Verification items for the finished model (mm, model axes). Round coordinates to 2 decimals unless told otherwise and drop trailing zeros. Write each loop counter-clockwise with the first axis right and the second up, starting at its lowest first coordinate (ties: lowest second). Pieces come first, ordered by that corner, then holes. Notation, with made-up numbers: (53.5, -13) - (81.5, -13) arc R17 cw to (81.5, 17) - close; hole circle Ø6 at (-3.75, 84). An arc over 180 degrees is marked (long way). Answer as a JSON object with one key per item and string values.
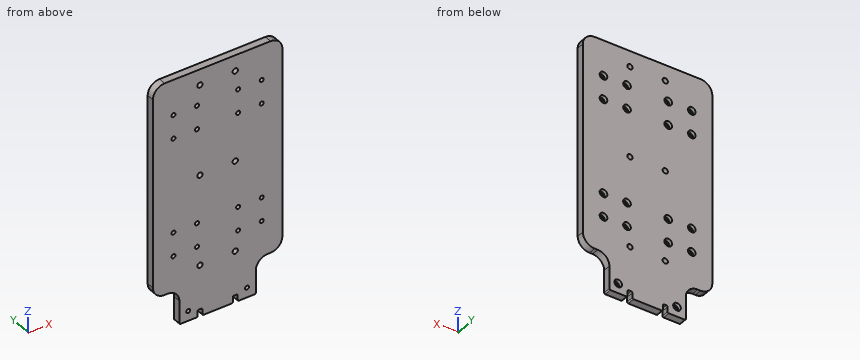
```python
from build123d import *

# Parameters (mm, degrees)
SKETCH1_W                      = 110
SKETCH1_H                      = 180
BOSS_EXTRUDE1_DEPTH            = 6.35
CBORE_START                    = 3.35
CBORE_FOR_M3_SHCS2_OUTLINE_R   = 3.25
CBORE_FOR_M3_SHCS2_DEPTH       = 3
CBORE_FOR_M3_SHCS2_2_OUTLINE_R = 1.7
CBORE_FOR_M3_SHCS2_2_DEPTH     = 3.35
M4_CLEARANCE_HOLE1_D           = 4.5
SKETCH6_W                      = 65
SKETCH6_H                      = 6.35
BOSS_EXTRUDE2_DEPTH            = 30
CBORE_FOR_M3_SHCS1_D           = 3.4
CBORE_FOR_M3_SHCS1_CBORE_D     = 6.5
CBORE_FOR_M3_SHCS1_CBORE_DEPTH = 3
FILLET2_R                      = 10
FILLET3_R                      = 10
SKETCH9_W                      = 4
SKETCH9_H                      = 6
CUT_EXTRUDE1_DEPTH             = 212.045782948
FILLET4_R                      = 1
FILLET5_R                      = 1
FILLET6_R                      = 1


# Read off the part's stored shape, not the designer's step: CBORE for M3 SHCS2
with BuildPart() as part:
    # Sketch1 → Boss-Extrude1 (new body)
    with BuildSketch(Plane(origin=(0, 0, 0), x_dir=(1, 0, 0), z_dir=(0, 1, 0))):
        with Locations((55, -90)):
            Rectangle(SKETCH1_W, SKETCH1_H)
    extrude(amount=BOSS_EXTRUDE1_DEPTH)

    # CBORE for M3 SHCS2 outline → CBORE for M3 SHCS2 (cut)
    with BuildSketch(Plane(origin=(0, 0, 0), x_dir=(1, 0, 0), z_dir=(0, 1, 0)).offset(CBORE_START)):
        with Locations((37.5, -150)):
            Circle(CBORE_FOR_M3_SHCS2_OUTLINE_R)
        with Locations((37.5, -130)):
            Circle(CBORE_FOR_M3_SHCS2_OUTLINE_R)
        with Locations((17.5, -130)):
            Circle(CBORE_FOR_M3_SHCS2_OUTLINE_R)
        with Locations((72.5, -150)):
            Circle(CBORE_FOR_M3_SHCS2_OUTLINE_R)
        with Locations((72.5, -130)):
            Circle(CBORE_FOR_M3_SHCS2_OUTLINE_R)
        with Locations((92.5, -130)):
            Circle(CBORE_FOR_M3_SHCS2_OUTLINE_R)
        with Locations((72.5, -30)):
            Circle(CBORE_FOR_M3_SHCS2_OUTLINE_R)
        with Locations((92.5, -50)):
            Circle(CBORE_FOR_M3_SHCS2_OUTLINE_R)
        with Locations((72.5, -50)):
            Circle(CBORE_FOR_M3_SHCS2_OUTLINE_R)
        with Locations((37.5, -30)):
            Circle(CBORE_FOR_M3_SHCS2_OUTLINE_R)
        with Locations((17.5, -50)):
            Circle(CBORE_FOR_M3_SHCS2_OUTLINE_R)
        with Locations((37.5, -50)):
            Circle(CBORE_FOR_M3_SHCS2_OUTLINE_R)
        with Locations((92.5, -150)):
            Circle(CBORE_FOR_M3_SHCS2_OUTLINE_R)
        with Locations((17.5, -30)):
            Circle(CBORE_FOR_M3_SHCS2_OUTLINE_R)
        with Locations((17.5, -150)):
            Circle(CBORE_FOR_M3_SHCS2_OUTLINE_R)
        with Locations((92.5, -30)):
            Circle(CBORE_FOR_M3_SHCS2_OUTLINE_R)
    extrude(amount=CBORE_FOR_M3_SHCS2_DEPTH, mode=Mode.SUBTRACT)

    # CBORE for M3 SHCS2 2 outline → CBORE for M3 SHCS2 2 (cut)
    with BuildSketch(Plane(origin=(0, 0, 0), x_dir=(1, 0, 0), z_dir=(0, 1, 0))):
        with Locations((37.5, -150)):
            Circle(CBORE_FOR_M3_SHCS2_2_OUTLINE_R)
        with Locations((37.5, -130)):
            Circle(CBORE_FOR_M3_SHCS2_2_OUTLINE_R)
        with Locations((17.5, -130)):
            Circle(CBORE_FOR_M3_SHCS2_2_OUTLINE_R)
        with Locations((72.5, -150)):
            Circle(CBORE_FOR_M3_SHCS2_2_OUTLINE_R)
        with Locations((72.5, -130)):
            Circle(CBORE_FOR_M3_SHCS2_2_OUTLINE_R)
        with Locations((92.5, -130)):
            Circle(CBORE_FOR_M3_SHCS2_2_OUTLINE_R)
        with Locations((72.5, -30)):
            Circle(CBORE_FOR_M3_SHCS2_2_OUTLINE_R)
        with Locations((92.5, -50)):
            Circle(CBORE_FOR_M3_SHCS2_2_OUTLINE_R)
        with Locations((72.5, -50)):
            Circle(CBORE_FOR_M3_SHCS2_2_OUTLINE_R)
        with Locations((37.5, -30)):
            Circle(CBORE_FOR_M3_SHCS2_2_OUTLINE_R)
        with Locations((17.5, -50)):
            Circle(CBORE_FOR_M3_SHCS2_2_OUTLINE_R)
        with Locations((37.5, -50)):
            Circle(CBORE_FOR_M3_SHCS2_2_OUTLINE_R)
        with Locations((92.5, -150)):
            Circle(CBORE_FOR_M3_SHCS2_2_OUTLINE_R)
        with Locations((17.5, -30)):
            Circle(CBORE_FOR_M3_SHCS2_2_OUTLINE_R)
        with Locations((17.5, -150)):
            Circle(CBORE_FOR_M3_SHCS2_2_OUTLINE_R)
        with Locations((92.5, -30)):
            Circle(CBORE_FOR_M3_SHCS2_2_OUTLINE_R)
    extrude(amount=CBORE_FOR_M3_SHCS2_2_DEPTH, mode=Mode.SUBTRACT)

    # M4 Clearance Hole1 (through all)
    with Locations(Plane.XZ):
        with Locations((70, 13.375), (70, 166.625), (40, 166.625), (70, 90), (40, 90), (40, 13.375)):
            Hole(M4_CLEARANCE_HOLE1_D / 2)

    # Sketch6 → Boss-Extrude2 (add)
    with BuildSketch(Plane(origin=(0, 0, 0), x_dir=(-1, 0, 0), z_dir=(0, 0, -1))):
        with Locations((-55, 3.175)):
            Rectangle(SKETCH6_W, SKETCH6_H)
    extrude(amount=BOSS_EXTRUDE2_DEPTH)

    # CBORE for M3 SHCS1 (through all)
    with Locations(Plane(origin=(0, 6.35, 0), x_dir=(1, 0, 0), z_dir=(0, 1, 0))):
        with Locations((30, 21.675), (80, 21.675)):
            CounterBoreHole(CBORE_FOR_M3_SHCS1_D / 2, CBORE_FOR_M3_SHCS1_CBORE_D / 2, CBORE_FOR_M3_SHCS1_CBORE_DEPTH)

    # Fillet2
    fillet2_edges = [part.edges().sort_by_distance(p)[0] for p in [
        (87.5, 3.175, 0),
        (22.5, 3.175, 0),
    ]]
    fillet(fillet2_edges, radius=FILLET2_R)

    # Fillet3
    fillet3_edges = [part.edges().sort_by_distance(p)[0] for p in [
        (0, 3.175, 0),
        (110, 3.175, 0),
        (110, 3.175, 180),
        (0, 3.175, 180),
    ]]
    fillet(fillet3_edges, radius=FILLET3_R)

    # Sketch9 → Cut-Extrude1 (cut, through all)
    with BuildSketch(Plane(origin=(0, 6.35, 0), x_dir=(1, 0, 0), z_dir=(0, 1, 0))):
        with Locations((70, 27)):
            Rectangle(SKETCH9_W, SKETCH9_H)
        with Locations((40, 27)):
            Rectangle(SKETCH9_W, SKETCH9_H)
    extrude(amount=-CUT_EXTRUDE1_DEPTH, mode=Mode.SUBTRACT)

    # Fillet4
    fillet4_edges = [part.edges().sort_by_distance(p)[0] for p in [
        (38, 3.175, -24),
        (42, 3.175, -24),
        (72, 3.175, -24),
        (68, 3.175, -24),
    ]]
    fillet(fillet4_edges, radius=FILLET4_R)

    # Fillet5
    fillet5_edges = [part.edges().sort_by_distance(p)[0] for p in [
        (38, 3.175, -30),
        (42, 3.175, -30),
        (72, 3.175, -30),
        (68, 3.175, -30),
    ]]
    fillet(fillet5_edges, radius=FILLET5_R)

    # Fillet6
    fillet6_edges = [part.edges().sort_by_distance(p)[0] for p in [
        (87.5, 3.175, -30),
        (22.5, 3.175, -30),
    ]]
    fillet(fillet6_edges, radius=FILLET6_R)


solid = part.part
```
Q1. Material ranges on line 1 along X through (y, z) = (2.5, 150); line 2 along Z through (x, y) = (70, 2) (3 decimals); line 3 along X through (y, z) = (1.25, -21), recorded low to high. Write a range as [from, to].
Geometry check:
{"line 1": "x = [0, 15.8], [19.2, 35.8], [39.2, 70.8], [74.2, 90.8], [94.2, 110]", "line 2": "z = [-24, 11.125], [15.625, 87.75], [92.25, 164.375], [168.875, 180]", "line 3": "x = [22.5, 28.44], [31.56, 78.44], [81.56, 87.5]"}
Q2. Section check B-B, the plane y = 5. State how many separate pieces and enclosed holes the cut face has, then the cut area to 3 significant figures.
Geometry check:
{"separate pieces": "1", "enclosed holes": "24", "area": "21,000 mm2"}
Q3. Section check A-A, the plane z = -5.5. Record the cut outline in (x, y).
Geometry check:
{"outline": "(21.43, 0) - (88.57, 0) - (88.57, 6.35) - (21.43, 6.35) - close"}
Q4. Gauge pin test, flat ends, axial feed: P1, Ø4, axis at x = 40, z = 13.375, coming from the -Y side; P2, Ø1.5, axis at x = 91.5, y = 5, coming from the -Z side; P3, Ø3, axis at x = 17, z = 151.5, coming from the +Y side; P4, Ø3, axis at x = 99, y = 2.5, coming from the -Z side. Record the tip position at first contact, or that the pin passes through.
Geometry check:
{"P1": "passes through", "P2": "stops at z = -2.62", "P3": "stops at y = 3.35", "P4": "stops at z = 0"}
